Geometry: final body of the model. Coordinates: model frame, mm. Face numbers are marked on the shaded views. A direction names the side the tool comes from. Give positions to 0.01 mm unless a question says otherwise; leave off trailing zeros. Order: outer loops, then holes, each group sorted by start corner. A loop starts at its lowest first (then second) coordinate and runs counter-clockwise, first axis right, second up. Notation, with made-up numbers: (81, -29) -> (125, -29) arc R18 cw to (125, 3) -> close; hole circle Ø1 at (14.25, 28). An arc over 180 degrees is marked (long way). Answer in a Markdown table with one row per item. Add a question column.
Q1. Line query: line 1 along X through (y, z) = (6, -37); line 2 along X through (y, z) = (3.55, -68.06); line 3 along X through (y, z) = (2.6, -77.2). Output: solid intervals per line, ascending. Write a range as from..to.
Q2. Cut plane D-D on x = 51.04. Return the cut outline in (y, z), and give its area (3 significant figures).
Q3. Set-up query: the marked faces 1 and 2. Return all of +Z, -Z, +X, -X, +Y, -Y with unobstructed straight access to the full face (end or side cutting, diameter ignored); none if empty.
Q4. Cut plane C-C on z = -46.5. Return the cut outline in (x, y).
Q5. Cut plane A-A on y = 6.75. Return the cut outline in (x, z), and give its area (3 significant figures).
Q6. Cut plane B-B on x = -1.7. Return the cut outline in (y, z).
Q7. Contact query for flat-ended pins moving along their axis: P1, Ø7.5, axis at x = 65.9, z = -19, coming from the +Y side; P2, Ø7, axis at x = -1.7, z = 1.7, coming from the +Y side; P3, Ø2.5, axis at y = 6.5, z = -43.5, coming from the +X side; P4, Ø3.5, axis at y = 6, z = -10, coming from the +X side. Output: stop coordinate, or through.
from build123d import *

# Parameters (mm, degrees)
SKETCH1_W           = 78.5
SKETCH1_H           = 75.5
BOSS_EXTRUDE1_DEPTH = 5
SKETCH2_W           = 10
SKETCH2_H           = 30
SKETCH2_W_2         = 4.083917928
SKETCH2_H_2         = 28.145920853
SKETCH2_H_3         = 8
BOSS_EXTRUDE2_DEPTH = 3
SKETCH6_R           = 2.15
BOSS_EXTRUDE3_DEPTH = 5
SKETCH3_R           = 1.6
CUT_EXTRUDE3_DEPTH  = 10
SKETCH5_R           = 3.25
CUT_EXTRUDE4_DEPTH  = 3
SKETCH9_W           = 78.5
SKETCH9_H           = 4
BOSS_EXTRUDE5_DEPTH = 4
FILLET2_R           = 10
FILLET3_R           = 10
FILLET4_R           = 10
FILLET5_R           = 10
FILLET6_R           = 10
FILLET7_R           = 10
FILLET8_R           = 10
FILLET9_R           = 10


with BuildPart() as part:
    # Sketch1 → Boss-Extrude1 (new body)
    with BuildSketch(Plane(origin=(0, 0, 0), x_dir=(1, 0, 0), z_dir=(0, 1, 0))):
        with Locations((39.25, 37.75)):
            Rectangle(SKETCH1_W, SKETCH1_H)
    extrude(amount=BOSS_EXTRUDE1_DEPTH)

    # Sketch2 → Boss-Extrude2 (add)
    with BuildSketch(Plane(origin=(0, 5, 0), x_dir=(1, 0, 0), z_dir=(0, 1, 0))):
        with Locations((15, 44.5)):
            Rectangle(SKETCH2_W, SKETCH2_H)
        with Locations((51.006989776, 48.944975154)):
            Rectangle(SKETCH2_W_2, SKETCH2_H_2)
        with Locations((43.5, 8)):
            Rectangle(SKETCH2_W, SKETCH2_H_3)
    extrude(amount=BOSS_EXTRUDE2_DEPTH)

    # Sketch6 → Boss-Extrude3 (add)
    # profile 1 of 4: a face of its own
    with BuildSketch(Plane(origin=(0, 0, 0), x_dir=(1, 0, 0), z_dir=(0, 1, 0))):
        with BuildLine():
            Line((0, 0), (0, 4.054128952))
            ThreePointArc((0, 4.054128952), (-5.942640687, -5.942640687), (4.054128952, 0))
            Line((4.054128952, 0), (0, 0))
        make_face()
        with Locations(Location((-1.7, -1.7, 0), (0, 0, 270))):
            Circle(SKETCH6_R, mode=Mode.SUBTRACT)
    # profile 2 of 4: a face of its own
    with BuildSketch(Plane(origin=(0, 0, 0), x_dir=(1, 0, 0), z_dir=(0, 1, 0))):
        with BuildLine():
            ThreePointArc((78.5, 4.054128952), (84.442640687, -5.942640687), (74.445871048, 0))
            Line((74.445871048, 0), (78.5, 0))
            Line((78.5, 0), (78.5, 4.054128952))
        make_face()
        with Locations(Location((80.2, -1.7, 0), (0, 0, 270))):
            Circle(SKETCH6_R, mode=Mode.SUBTRACT)
    # profile 3 of 4: a face of its own
    with BuildSketch(Plane(origin=(0, 0, 0), x_dir=(1, 0, 0), z_dir=(0, 1, 0))):
        with BuildLine():
            ThreePointArc((0, 71.445871048), (-5.942640687, 81.442640687), (4.054128952, 75.5))
            Line((4.054128952, 75.5), (0, 75.5))
            Line((0, 75.5), (0, 71.445871048))
        make_face()
        with Locations(Location((-1.7, 77.2, 0), (0, 0, 270))):
            Circle(SKETCH6_R, mode=Mode.SUBTRACT)
    # profile 4 of 4: a face of its own
    with BuildSketch(Plane(origin=(0, 0, 0), x_dir=(1, 0, 0), z_dir=(0, 1, 0))):
        with BuildLine():
            Line((78.5, 75.5), (78.5, 71.445871048))
            ThreePointArc((78.5, 71.445871048), (84.442640687, 81.442640687), (74.445871048, 75.5))
            Line((74.445871048, 75.5), (78.5, 75.5))
        make_face()
        with Locations(Location((80.2, 77.2, 0), (0, 0, 270))):
            Circle(SKETCH6_R, mode=Mode.SUBTRACT)
    extrude(amount=BOSS_EXTRUDE3_DEPTH)

    # Sketch3 → Cut-Extrude3 (cut)
    with BuildSketch(Plane(origin=(0, 5, 0), x_dir=(1, 0, 0), z_dir=(0, 1, 0))):
        with Locations(Location((7.54, 17.25, 0), (0, 0, 270))):
            Circle(SKETCH3_R)
        with Locations(Location((55.86, 16, 0), (0, 0, 270))):
            Circle(SKETCH3_R)
        with Locations(Location((22.87, 68.06, 0), (0, 0, 270))):
            Circle(SKETCH3_R)
        with Locations(Location((51.04, 68.06, 0), (0, 0, 270))):
            Circle(SKETCH3_R)
        with Locations(Location((65.9, 19, 0), (0, 0, 270))):
            Circle(SKETCH3_R)
    extrude(amount=-CUT_EXTRUDE3_DEPTH, mode=Mode.SUBTRACT)

    # Sketch5 → Cut-Extrude4 (cut)
    with BuildSketch(Plane.XZ):
        with Locations(Location((7.54, -17.25, 0), (0, 0, 270))):
            Circle(SKETCH5_R)
        with Locations(Location((55.86, -16, 0), (0, 0, 270))):
            Circle(SKETCH5_R)
        with Locations(Location((22.87, -68.06, 0), (0, 0, 270))):
            Circle(SKETCH5_R)
        with Locations(Location((51.04, -68.06, 0), (0, 0, 270))):
            Circle(SKETCH5_R)
        with Locations(Location((65.9, -19, 0), (0, 0, 270))):
            Circle(SKETCH5_R)
    extrude(amount=-CUT_EXTRUDE4_DEPTH, mode=Mode.SUBTRACT)

    # Sketch9 → Boss-Extrude5 (add)
    with BuildSketch(Plane(origin=(0, 5, 0), x_dir=(1, 0, 0), z_dir=(0, 1, 0))):
        with Locations((39.25, 2)):
            Rectangle(SKETCH9_W, SKETCH9_H)
    extrude(amount=BOSS_EXTRUDE5_DEPTH)

    # Fillet2
    fillet2_edges = [part.edges().sort_by_distance(p)[0] for p in [
        (4.054128952, 2.5, 0),
    ]]
    fillet(fillet2_edges, radius=FILLET2_R)

    # Fillet3
    fillet3_edges = [part.edges().sort_by_distance(p)[0] for p in [
        (74.445871048, 2.5, 0),
    ]]
    fillet(fillet3_edges, radius=FILLET3_R)

    # Fillet4
    fillet4_edges = [part.edges().sort_by_distance(p)[0] for p in [
        (78.5, 2.5, -4.054128952),
    ]]
    fillet(fillet4_edges, radius=FILLET4_R)

    # Fillet5
    fillet5_edges = [part.edges().sort_by_distance(p)[0] for p in [
        (78.5, 2.5, -71.445871048),
    ]]
    fillet(fillet5_edges, radius=FILLET5_R)

    # Fillet6
    fillet6_edges = [part.edges().sort_by_distance(p)[0] for p in [
        (74.445871048, 2.5, -75.5),
    ]]
    fillet(fillet6_edges, radius=FILLET6_R)

    # Fillet7
    fillet7_edges = [part.edges().sort_by_distance(p)[0] for p in [
        (4.054128952, 2.5, -75.5),
    ]]
    fillet(fillet7_edges, radius=FILLET7_R)

    # Fillet8
    fillet8_edges = [part.edges().sort_by_distance(p)[0] for p in [
        (0, 2.5, -71.445871048),
    ]]
    fillet(fillet8_edges, radius=FILLET8_R)

    # Fillet9
    fillet9_edges = [part.edges().sort_by_distance(p)[0] for p in [
        (0, 2.5, -4.054128952),
    ]]
    fillet(fillet9_edges, radius=FILLET9_R)


solid = part.part
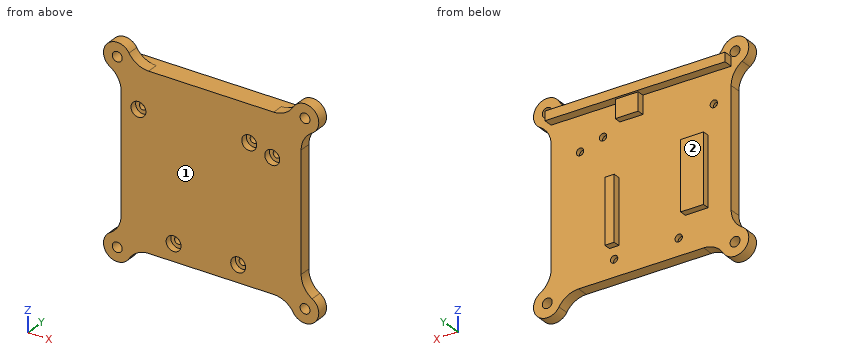
Completed:
| question | item | result |
|---|---|---|
| 1 | line 1 | x = 10..20, 48.97..53.05 |
| 1 | line 2 | x = -1.09..21.27, 24.47..49.44, 52.64..79.59 |
| 1 | line 3 | x = -7.7..-3.85, 0.45..6.4, 72.1..78.05, 82.35..86.2 |
| 2 | outline | (0, -75.5) -> (5, -75.5) -> (5, -69.66) -> (3, -69.66) -> (3, -71.31) -> (0, -71.31) -> close; (0, -64.81) -> (3, -64.81) -> (3, -66.46) -> (5, -66.46) -> (5, -63.02) -> (8, -63.02) -> (8, -34.87) -> (5, -34.87) -> (5, -4) -> (9, -4) -> (9, 0) -> (0, 0) -> close |
| 2 | area | 452 mm² |
| 3 | face 1 | +Z, -Z, +X, -X, -Y |
| 3 | face 2 | -Z, +X, -X, +Y |
| 4 | outline | (0, 0) -> (78.5, 0) -> (78.5, 5) -> (53.05, 5) -> (53.05, 8) -> (48.97, 8) -> (48.97, 5) -> (20, 5) -> (20, 8) -> (10, 8) -> (10, 5) -> (0, 5) -> close |
| 5 | outline | (0, -4) -> (38.5, -4) -> (38.5, -12) -> (48.5, -12) -> (48.5, -4) -> (78.5, -4) -> (78.5, 0) -> (0, 0) -> close; (10, -59.5) -> (20, -59.5) -> (20, -29.5) -> (10, -29.5) -> close; (48.97, -63.02) -> (53.05, -63.02) -> (53.05, -34.87) -> (48.97, -34.87) -> close |
| 5 | area | 809 mm² |
| 6 | outline | (0, -83.2) -> (5, -83.2) -> (5, -79.35) -> (0, -79.35) -> close; (0, -75.05) -> (5, -75.05) -> (5, -69.1) -> (0, -69.1) -> close; (0, -6.4) -> (5, -6.4) -> (5, -0.45) -> (0, -0.45) -> close; (0, 3.85) -> (5, 3.85) -> (5, 7.7) -> (0, 7.7) -> close |
| 7 | P1 | stops at y = 5 |
| 7 | P2 | stops at y = 9 |
| 7 | P3 | stops at x = 53.05 |
| 7 | P4 | stops at x = 79.1 |
